from build123d import *

# Parameters (mm, degrees)
F3_W     = 94
F3_H     = 34
F4_DEPTH = 50


with BuildPart() as f4:
    # F3 (on Front) → F4 (new body, symmetric)
    with BuildSketch(Plane.XZ):
        with BuildLine():
            ThreePointArc((-19.2521204937, -49.7380952381), (-18.6663340561, -51.1523088005), (-17.2521204937, -51.7380952381))
            Line((-17.2521204937, -51.7380952381), (78.7478795063, -51.7380952381))
            ThreePointArc((78.7478795063, -51.7380952381), (80.1620930687, -51.1523088005), (80.7478795063, -49.7380952381))
            Line((80.7478795063, -49.7380952381), (80.7478795063, -13.7380952381))
            ThreePointArc((80.7478795063, -13.7380952381), (80.1620930687, -12.3238816757), (78.7478795063, -11.7380952381))
            Line((78.7478795063, -11.7380952381), (-17.2521204937, -11.7380952381))
            ThreePointArc((-17.2521204937, -11.7380952381), (-18.6663340561, -12.3238816757), (-19.2521204937, -13.7380952381))
            Line((-19.2521204937, -13.7380952381), (-19.2521204937, -49.7380952381))
        make_face()
        with Locations((30.7478795063, -31.7380952381)):
            Rectangle(F3_W, F3_H, mode=Mode.SUBTRACT)
    extrude(amount=F4_DEPTH, both=True)


with BuildPart() as f5_1:
    # F5: copy of F4
    add(f4.part)


solid = f4.part
Check sheet for the modelled part. Datum: model origin and axes. Units: mm. A direction names the side the tool comes from. Give positions to 0.01 mm unless a question says otherwise; leave off trailing zeros. Write each loop counter-clockwise with the first axis right and the second up, starting at its lowest first coordinate (ties: lowest second). Pieces come first, ordered by that corner, then holes. Notation, with made-up numbers: M -16.5,-7 L -5.5,-7 A25 ccw -5.5,29 Z; hole C 67.25,70 d10. An arc over 180 degrees is marked long. Use one line per item in the form item = value.
(1) Section check C-C on x = 6.5. Record the boundary of the cut face in (y, z), plus the area to 3 significant figures.
Answer block:
outline = M -50,-51.74 L 50,-51.74 L 50,-48.74 L -50,-48.74 Z; M -50,-14.74 L 50,-14.74 L 50,-11.74 L -50,-11.74 Z
area = 600 mm2
(2) Section check B-B on y = -14.5. Record the boundary of the cut face in (x, z).
Answer block:
outline = M -19.25,-49.74 A2 ccw -17.25,-51.74 L 78.75,-51.74 A2 ccw 80.75,-49.74 L 80.75,-13.74 A2 ccw 78.75,-11.74 L -17.25,-11.74 A2 ccw -19.25,-13.74 Z; hole M -16.25,-48.74 L 77.75,-48.74 L 77.75,-14.74 L -16.25,-14.74 Z
(3) Material ranges on line 1 along Z through (x, y) = (74, -17.5); line 2 along X through (y, z) = (6, -36.5); line 3 along X through (y, z) = (28.5, -50), recorded low to high.
Answer block:
line_1 = -51.74 to -48.74, -14.74 to -11.74
line_2 = -19.25 to -16.25, 77.75 to 80.75
line_3 = -19.23 to 80.73
(4) Section check A-A on z = -46. Record the boundary of the cut face in (x, y), plus the area to 3 significant figures.
Answer block:
outline = M -19.25,-50 L -16.25,-50 L -16.25,50 L -19.25,50 Z; M 77.75,-50 L 80.75,-50 L 80.75,50 L 77.75,50 Z
area = 600 mm2
(5) Draft check along Z on faces 3 (the flat face through (-16.252, -1, -32)), 4 (the flat face through (80.748, -1, -32)), 5 (the flat face through (30, -1, -51.738)), 6 (the flat face through (31, -1, -11.738)). Enter one of: pulls with the +Z half, pulls with the -Z half, needs draft (parallel to the pull), parting line crosses it, or undercut.
Answer block:
face_3 = undercut
face_4 = needs draft
face_5 = pulls with the -Z half
face_6 = pulls with the +Z half
(6) Tool access check on faces 1 (the flat face through (27, -50, -49)), 2 (the flat face through (77.748, -1, -32)). Record the directions out of +Z, -Z, +X, -X, +Y, -Y that give a thin tool (end or side, any length) a straight path to the whole face; none if there is none.
Answer block:
face_1 = +Z, -Z, +X, -X, -Y
face_2 = +Y, -Y
